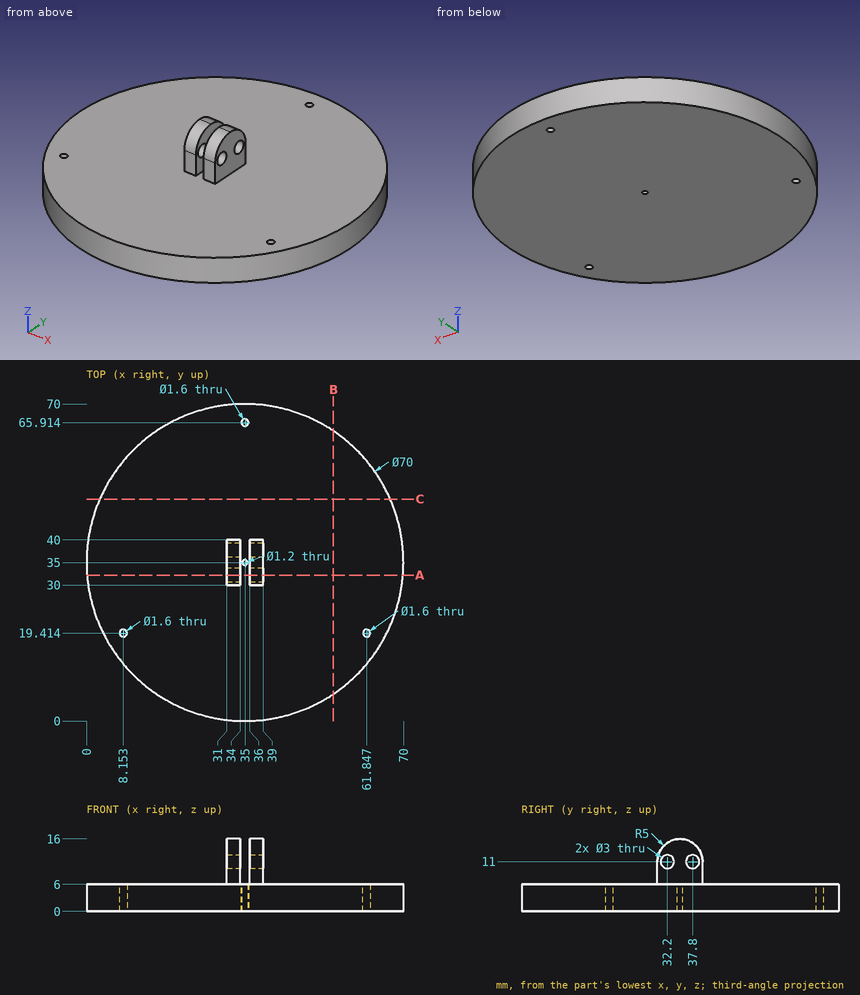
Check sheet for the drawn part. Datum: minimum x, y, z corner. Units: mm. Coordinates: 2 decimals unless noted, no trailing zeros. Loops run counter-clockwise (first coordinate to the right, second up) from the corner with the lowest first, then second, coordinate; pieces in that order, holes last. Notation, with made-up numbers: (67.25, 42) -> (119.25, 42) arc R11 cw to (119.25, 52) -> close; hole circle Ø1 at (8.25, 19.25). An arc over 180 degrees is marked (long way). Answer as a JSON object with one key per item and string values. Group by question number.
Item 1: Sectioned sample at A-A on y = 32.2. Record the boundary of the cut face in (x, z).
Item 2: Sectioned sample at C-C on y = 49. Record the boundary of the cut face in (x, z), plus the area to 3 significant figures.
Item 3: Scan lines: probe 1 along Z at (x, y) = (33, 59); probe 2 along X at (y, z) = (35.5, 1.5) (1 decimal); probe 3 along Z at (x, y) = (37, 32). Record each from-to range of solid material in increasing order.
Item 4: Depth check by flat-ended pin: pin 1 (3 mm diameter, centred on y = 37.5, z = 9.5, fed in from -X); pin 2 (2.5 mm diameter, centred on x = 32.5, z = 9, fed in from -Y); pin 3 (5 mm diameter, centred on x = 59.5, y = 16, fed in from +Z). Enter the tip coordinate at first touch or a pass-through.
Item 5: Sectioned sample at B-B on x = 54.5. Record the boundary of the cut face in (y, z) (1 decimal), plus the area to 3 significant figures.
Evaluation:
{
 "1": {"outline": "(0.11, 0) -> (69.89, 0) -> (69.89, 6) -> (39, 6) -> (39, 9.5) -> (36, 9.5) -> (36, 6) -> (34, 6) -> (34, 9.5) -> (31, 9.5) -> (31, 6) -> (0.11, 6) -> close; (31, 12.5) -> (34, 12.5) -> (34, 15.14) -> (31, 15.14) -> close; (36, 12.5) -> (39, 12.5) -> (39, 15.14) -> (36, 15.14) -> close"},
 "2": {"outline": "(2.92, 0) -> (67.08, 0) -> (67.08, 6) -> (2.92, 6) -> close", "area": "385 mm²"},
 "3": {"probe 1": "z = 0 to 6", "probe 2": "x = 0 to 34.7, 35.3 to 70", "probe 3": "z = 0 to 9.51, 12.49 to 15"},
 "4": {"pin 1": "stops at x = 31", "pin 2": "stops at y = 30", "pin 3": "stops at z = 6"},
 "5": {"outline": "(5.9, 0) -> (64.1, 0) -> (64.1, 6) -> (5.9, 6) -> close", "area": "349 mm²"}
}
